Autodesk Inventor part; units mm, degrees
ref_plane "YZ Plane" through (0, 0, 0) normal (1, 0, 0) x (0, 1, 0)
ref_plane "XZ Plane" through (0, 0, 0) normal (0, 1, 0) x (-1, 0, 0)
ref_plane "XY Plane" through (0, 0, 0) normal (0, 0, 1) x (1, 0, 0)
sketch "Náčrt6" plane through (0, 0, 0) normal (0, 1, 0) x (-1, 0, 0)
  line L0 (-7.5, 5) -> (7.5, 5)
  line L1 (7.5, 5) -> (7.5, -5)
  line L2 (7.5, -5) -> (-7.5, -5)
  line L3 (-7.5, -5) -> (-7.5, 5)
  line L4 (-7.5, 5) -> (7.5, -5) construction
  line L5 (7.5, 5) -> (-7.5, -5) construction
  point P0 (0, 0)
  dimension "d10" = 15
  dimension "d11" = 10
extrude "Vysunutí6" add sketch "Náčrt6" along normal blind 7
sketch "Náčrt7" plane through (0, 0, 0) normal (0, 0, 1) x (1, 0, 0)
  line L0 (0, 8.4) -> (0, -1.4)
  line L1 (-10.5, 0) -> (10.5, 0)
  line L2 (-4.75, 7) -> (4.75, 7)
  line L3 (4.75, 7) -> (4.75, 5)
  line L4 (3.75, 4) -> (-3.75, 4)
  line L5 (-4.75, 5) -> (-4.75, 7)
  line L6 (7.5, 7) -> (-7.5, 7)
  line L7 (-4.75, 5) -> (-3.75, 4)
  line L8 (3.75, 4) -> (4.75, 5)
  point P0 (0, 0)
  point P1 (4.75, 4)
  point P2 (-4.75, 4)
  dimension "d14" = 9.5
  dimension "d15" = 3
  dimension "d16" = 1
  dimension "d17" = 1
  dimension "d18" = 1
  dimension "d19" = 1
extrude "Vysunutí7" cut sketch "Náčrt7" against normal through all both and the other way through all
sketch "Náčrt8" plane through (7.5, 0, 5) normal (1, 0, 0) x (0, 0, -1)
  line L0 (0, 0) -> (10, 0)
  line L1 (2.5, 0) -> (7.5, 0)
  line L2 (7.5, 0) -> (7.5, 6)
  line L3 (7.5, 6) -> (2.5, 6)
  line L4 (2.5, 6) -> (2.5, 0)
  line L5 (-2, 0) -> (12, 0)
  line L6 (5, -1.4) -> (5, 8.4)
  point P0 (5, 0)
  dimension "d22" = 5
  dimension "d23" = 6
extrude "Vysunutí8" cut sketch "Náčrt8" against normal blind 3
mirror "Zrcadlit1" about plane through (0, 0, 0) normal (1, 0, 0) of "Vysunutí8"
sketch "Náčrt9" plane through (4.5, 0, 5) normal (1, 0, 0) x (0, 0, -1)
  line L0 (2.5, 4.75) -> (7.5, 4.75)
  line L1 (2.5, 0) -> (2.5, 4.75)
  line L2 (7.5, 0) -> (2.5, 0)
  line L3 (7.5, 4.75) -> (7.5, 0)
  line L4 (10, 4) -> (0, 4)
  point P0 (5, 0)
  point P1 (2.5, 4)
  point P2 (7.5, 4)
extrude "Vysunutí9" cut sketch "Náčrt9" against normal through all contours L0 L3 L4 L1
sketch "Náčrt10" plane through (-3.75, 4, -5) normal (0, 1, 0) x (1, 0, 0)
  point P0 (3.75, -5)
hole "Díra1" at (0, 4, 0) direction (0, -1, 0) diameter 3.7 end through all counterbore diameter 7 counterbore depth 2.5
fillet "Zaoblení1" radius 1 4 edges at (7.5, 3.5, -5) (7.5, 3.5, 5) (-7.5, 3.5, -5) (-7.5, 3.5, 5)
equation "\"Milimetr\" = 1"
properties part number "Příchytka pásků, pro M3, přírodní bílá" material "Plast, neprůhledný bílý"
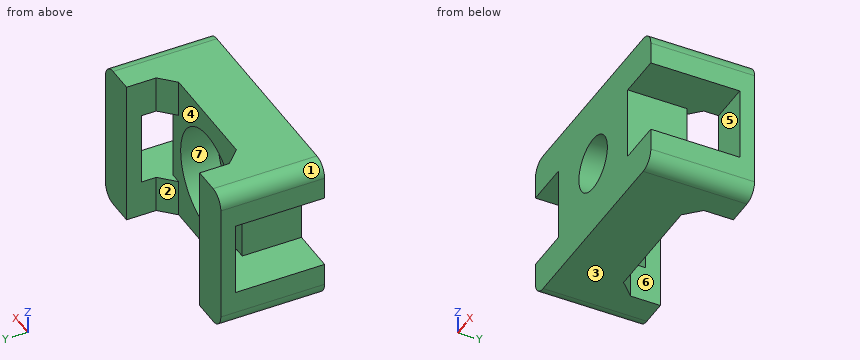
Build history of the part. All positions in model axes, mm. Face numbers are marked on the shaded views. A direction names the side the tool comes from. Round coordinates to 2 decimals unless told otherwise and drop trailing zeros. Write each loop counter-clockwise with the first axis right and the second up, starting at its lowest first coordinate (ties: lowest second). Pieces come first, ordered by that corner, then holes. Notation, with made-up numbers: M -2,-21.75 L 22,-21.75 A24 cw 22,12.25 Z; hole C 61.5,70 d1. An arc over 180 degrees is marked long. Answer as a JSON object with one key per item and string values. Group by question number.
(1) Mould opens along Z. For the marked faces 1, 2, 3 and 4 say: pulls with the +Z half, pulls with the -Z half, needs draft (parallel to the pull), parting line crosses it, or undercut.
(2) Drill centre lines: L1, parallel to Z at x = 0, y = 0.8; L2, parallel to X at y = 3.35, z = 0; L3, parallel to X at y = 0.55, z = 0. Where is each one in solid material? Low to high.
(3) Cut at A-A (x = 0). Give the cut face in (y, z), and give its area (4 significant figures).
(4) Cut at D-D (y = 3.5). Give the cut face in (x, z).
(5) Which spindle directions (+Z, -Z, +X, -X, +Y, -Y) get a long thin tool onto all of the face, cutting with end or side? Do the marked faces 5, 6 and 7. Say none if no direction does.
(6) Cut at C-C (y = 5.25). Give the cut face in (x, z).
(7) Cut at B-B (z = 0). Give the cut face in (x, y), and give its area (4 significant figures).
(8) Flat gauge pins, fed straight in: pin 1 (3 mm diameter, centred on y = 3, z = 0, fed in from +X); pin 2 (3 mm diameter, centred on x = 0, z = 1.5, fed in from +Y); pin 3 (0.8 mm diameter, centred on x = -6.5, z = 1, fed in from -Y); pin 4 (3.5 mm diameter, centred on x = 0, z = 0, fed in from -Y). Where does each tip first touch, or does it go through?
Responses:
{
 "1": {"face 1": "pulls with the +Z half", "face 2": "needs draft", "face 3": "pulls with the -Z half", "face 4": "undercut"},
 "2": {"L1": "z = -5 to -1.85, 1.85 to 5", "L2": "x = -4.5 to -3.5, 3.5 to 4.5", "L3": "x = -4.5 to -1.85, 1.85 to 4.5"},
 "3": {"outline": "M 0,-5 L 4,-5 L 4,-3.5 L 1.5,-3.5 L 1.5,-1.85 L 0,-1.85 Z; M 0,1.85 L 1.5,1.85 L 1.5,3.5 L 4,3.5 L 4,5 L 0,5 Z", "area": "16.95 mm2"},
 "4": {"outline": "M -7.5,-4 A1 ccw -6.5,-5 L 6.5,-5 A1 ccw 7.5,-4 L 7.5,-2.5 L 4.5,-2.5 L 4.5,2.5 L 7.5,2.5 L 7.5,4 A1 ccw 6.5,5 L -6.5,5 A1 ccw -7.5,4 L -7.5,2.5 L -4.5,2.5 L -4.5,-2.5 L -7.5,-2.5 Z; hole C 0,0 d7"},
 "5": {"face 5": "+X, -X, -Y", "face 6": "+Z, -Z, +Y", "face 7": "+Y"},
 "6": {"outline": "M -7.5,-4 A1 ccw -6.5,-5 L -4.75,-5 L -4.75,-2.5 L -7.5,-2.5 Z; M -7.5,2.5 L -4.75,2.5 L -4.75,5 L -6.5,5 A1 ccw -7.5,4 Z; M 4.75,-5 L 6.5,-5 A1 ccw 7.5,-4 L 7.5,-2.5 L 4.75,-2.5 Z; M 4.75,2.5 L 7.5,2.5 L 7.5,4 A1 ccw 6.5,5 L 4.75,5 Z"},
 "7": {"outline": "M -7.5,6 L -4.75,6 L -4.75,7 L -7.5,7 Z; M -4.5,0 L -1.85,0 L -1.85,1.5 L -3.5,1.5 L -3.5,4 L -4.5,4 Z; M 1.85,0 L 4.5,0 L 4.5,4 L 3.5,4 L 3.5,1.5 L 1.85,1.5 Z; M 4.75,6 L 7.5,6 L 7.5,7 L 4.75,7 Z", "area": "18.45 mm2"},
 "8": {"pin 1": "stops at x = 4.5", "pin 2": "stops at y = 1.5", "pin 3": "stops at y = 6", "pin 4": "passes through"}
}
